Geometry check sheet. Reference: the model listing, model coordinates, mm. Give positions to 0.01 mm unless a question says otherwise; leave off trailing zeros. Loops run counter-clockwise (first coordinate to the right, second up) from the corner with the lowest first, then second, coordinate; pieces in that order, holes last. Notation, with made-up numbers: (34.25, 80) -> (43.25, 80) arc R16 cw to (43.25, 99) -> close; hole circle Ø4 at (24.5, 75). An arc over 180 degrees is marked (long way). Write item = value, one per line. Start each with the question number.
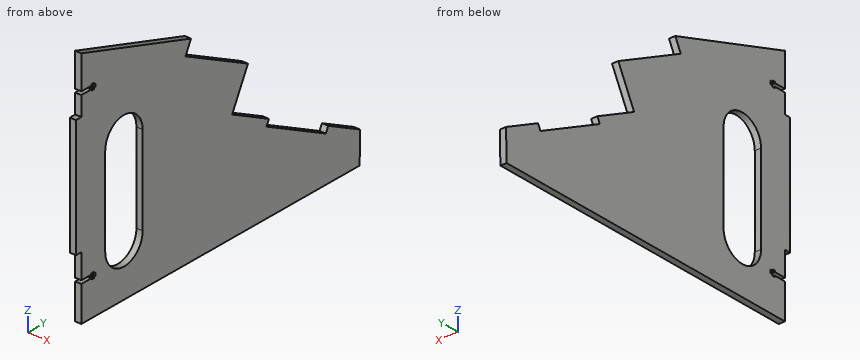
```python
from build123d import *

# Parameters (mm, degrees)
BOSS_EXTRUDE1_DEPTH = 6
CUT_EXTRUDE1_DEPTH  = 6
SKETCH3_W           = 6
SKETCH3_H           = 113
BOSS_EXTRUDE2_DEPTH = 6
SKETCH4_W           = 3.1
SKETCH4_H           = 16
CUT_EXTRUDE2_DEPTH  = 6
SKETCH5_W           = 5.5
SKETCH5_H           = 2.8
CUT_EXTRUDE3_DEPTH  = 6


with BuildPart() as part:
    # Sketch1 → Boss-Extrude1 (new body)
    with BuildSketch(Plane(origin=(0, 0, 0), x_dir=(0, 0, -1), z_dir=(1, 0, 0))):
        Polygon((42.307983077, 123.832979907), (2.448355916, 0.258483339), (228.768209888, 0.258483339), (228.768209888, 313.843147788), (198.909979532, 314.531209333), (180.529620903, 278.442257884), (185.876132229, 275.719241791), (151.838431063, 208.887850219), (146.491919737, 211.610866313), (125.388545015, 170.175403538), (90.368895831, 188.011158949), (54.515850604, 117.615426494), align=None)
    extrude(amount=BOSS_EXTRUDE1_DEPTH)

    # Sketch2 → Cut-Extrude1 (cut)
    with BuildSketch(Plane(origin=(6, 0, 0), x_dir=(0, 0, -1), z_dir=(1, 0, 0))):
        with BuildLine():
            Line((95.286629817, 69.348811068), (179.963244622, 69.348811068))
            ThreePointArc((179.963244622, 69.348811068), (201.051431087, 48.260624604), (179.963244622, 27.172438139))
            Line((179.963244622, 27.172438139), (95.286629817, 27.172438139))
            ThreePointArc((95.286629817, 27.172438139), (74.198443353, 48.260624604), (95.286629817, 69.348811068))
        make_face()
    extrude(amount=-CUT_EXTRUDE1_DEPTH, mode=Mode.SUBTRACT)

    # Sketch3 → Boss-Extrude2 (add)
    with BuildSketch(Plane.XZ.offset(-0.258483339)):
        with Locations((3, -112.268209888)):
            Rectangle(SKETCH3_W, SKETCH3_H)
    extrude(amount=BOSS_EXTRUDE2_DEPTH)

    # Sketch4 → Cut-Extrude2 (cut)
    with BuildSketch(Plane(origin=(6, 0, 0), x_dir=(0, 0, -1), z_dir=(1, 0, 0))):
        with Locations((35.768209888, 8.258483339)):
            Rectangle(SKETCH4_W, SKETCH4_H)
        with Locations((193.768209888, 8.258483339)):
            Rectangle(SKETCH4_W, SKETCH4_H)
    extrude(amount=-CUT_EXTRUDE2_DEPTH, mode=Mode.SUBTRACT)

    # Sketch5 → Cut-Extrude3 (cut)
    with BuildSketch(Plane(origin=(6, 0, 0), x_dir=(0, 0, -1), z_dir=(1, 0, 0))):
        with Locations((35.768209888, 12.858483339)):
            Rectangle(SKETCH5_W, SKETCH5_H)
        with Locations((193.768209888, 12.858483339)):
            Rectangle(SKETCH5_W, SKETCH5_H)
    extrude(amount=-CUT_EXTRUDE3_DEPTH, mode=Mode.SUBTRACT)


solid = part.part
```
1) Thickness scan on line 1 (Y direction, x = 1.6, z = -80.5); line 2 (Z direction, x = 4.9, y = 176); line 3 (Y direction, x = 3.15, z = -202). Record the ranges inside material, lowest first.
2) Section check B-B (z = -156). Enter the section's corners in (x, y).
3) Depth check by flat-ended pin: pin 1 Ø0.6 at (x, y) = (4, 15.5) entering from +Z; pin 2 Ø1.8 at (x, z) = (4, -23) entering from -Y; pin 3 Ø3 at (x, y) = (2, 13.5) entering from +Z. Enter the tip coordinate at first touch or a pass-through.
4) Section check A-A (y = 50). Enter the section's corners in (x, z), plus the area to 3 significant figures.
5) Section check C-C (z = -207). Enter the section's corners in (x, y).
6) Section check D-D (y = 141). Enter the section's corners in (x, z), plus the area to 3 significant figures.
Check result:
q1.line_1 = -5.74 to 33.23, 63.3 to 168.63
q1.line_2 = -228.77 to -128.36, -113.95 to -84.25
q1.line_3 = 0.26 to 314.46
q2.outline = (0, -5.74) -> (6, -5.74) -> (6, 27.17) -> (0, 27.17) -> close; (0, 69.35) -> (6, 69.35) -> (6, 217.06) -> (0, 217.06) -> close
q3.pin_1 = -7.27
q3.pin_2 = 0.26
q3.pin_3 = -6.24
q4.outline = (0, -228.77) -> (6, -228.77) -> (6, -200.98) -> (0, -200.98) -> close; (0, -74.27) -> (6, -74.27) -> (6, -18.49) -> (0, -18.49) -> close
q4.area = 501 mm2
q5.outline = (0, 0.26) -> (6, 0.26) -> (6, 314.34) -> (0, 314.34) -> close
q6.outline = (0, -228.77) -> (6, -228.77) -> (6, -66.43) -> (0, -66.43) -> close
q6.area = 974 mm2
